Input: part model. Units: mm. Frame: model coordinates. Face numbers are marked on the shaded views. A direction names the side the tool comes from. Give positions to 0.01 mm unless a question says otherwise; leave off trailing zeros. Order: outer loops, then holes, each group sorted by start corner. A loop starts at its lowest first (then second) coordinate and runs counter-clockwise, first axis right, second up. Notation, with made-up numbers: (-18, 12) - (-7, 12) arc R16 cw to (-7, 31) - close; hole circle Ø10 at (30, -19.5). An arc over 180 degrees is marked (long way). Use a Markdown table: item, result.
from build123d import *

# Parameters (mm, degrees)
SKETCH_1_W           = 116
SKETCH_1_H           = 70
EXTRUDE_1_DEPTH      = 66
SKETCH_2_W           = 110
SKETCH_2_H           = 60
CUT_EXTRUDE_1_DEPTH  = 67
CUT_EXTRUDE_2_REACH  = 118
SKETCH_3_W           = 65
SKETCH_3_H           = 13
CUT_EXTRUDE_3_REACH  = 118
SKETCH_4_W           = 65
SKETCH_4_H           = 9.8
CUT_EXTRUDE_4_REACH  = 68
SKETCH_5_W           = 92
SKETCH_5_H           = 3
CUT_EXTRUDE_5_REACH  = 118
SKETCH_6_W           = 33
SKETCH_6_H           = 42
SKETCH_7_W           = 92
SKETCH_7_H           = 3
CUT_EXTRUDE_6_DEPTH  = 67
CUT_EXTRUDE_7_DEPTH  = 4
CUT_EXTRUDE_8_DEPTH  = 4
CUT_EXTRUDE_9_DEPTH  = 4
CUT_EXTRUDE_10_DEPTH = 4
CUT_EXTRUDE_11_DEPTH = 4
CUT_EXTRUDE_12_REACH = 118
CUT_EXTRUDE_13_DEPTH = 67
CUT_EXTRUDE_14_DEPTH = 67
CUT_EXTRUDE_15_DEPTH = 67
CUT_EXTRUDE_16_DEPTH = 67
CUT_EXTRUDE_17_DEPTH = 67
CUT_EXTRUDE_18_REACH = 68
CUT_EXTRUDE_19_REACH = 118
CUT_EXTRUDE_20_DEPTH = 67
FILLET_1_R           = 2
SKETCH_22_W          = 129.509915456
SKETCH_22_H          = 79.224014217
CUT_EXTRUDE_22_DEPTH = 30
SKETCH_23_W          = 92
SKETCH_23_H          = 66
CUT_EXTRUDE_23_DEPTH = 3
CUT_EXTRUDE_24_DEPTH = 8


with BuildPart() as part:
    # 스케치1 → 보스-돌출1 (new body)
    with BuildSketch(Plane.XZ.offset(33)):
        with Locations((0, 35)):
            Rectangle(SKETCH_1_W, SKETCH_1_H)
    extrude(amount=-EXTRUDE_1_DEPTH)

    # 스케치2 → 컷-돌출1 (cut)
    with BuildSketch(Plane.XY.offset(70)):
        Rectangle(SKETCH_2_W, SKETCH_2_H)
    extrude(amount=-CUT_EXTRUDE_1_DEPTH, mode=Mode.SUBTRACT)

    # 스케치3 → 컷-돌출2 (cut, up to next)
    with BuildSketch(Plane.ZY.offset(58), mode=Mode.PRIVATE) as cut_extrude_2_sk1:
        with Locations((37.5, 14.5)):
            Rectangle(SKETCH_3_W, SKETCH_3_H)
    cut_extrude_2_tool1 = extrude(cut_extrude_2_sk1.sketch, amount=-CUT_EXTRUDE_2_REACH, mode=Mode.PRIVATE) & part.part
    add(cut_extrude_2_tool1.solids().sort_by_distance((-58, 14.5, 37.5))[0], mode=Mode.SUBTRACT)

    # 스케치4 → 컷-돌출3 (cut, up to next)
    with BuildSketch(Plane.ZY.offset(58), mode=Mode.PRIVATE) as cut_extrude_3_sk1:
        with Locations((37.5, -16.3)):
            Rectangle(SKETCH_4_W, SKETCH_4_H)
    cut_extrude_3_tool1 = extrude(cut_extrude_3_sk1.sketch, amount=-CUT_EXTRUDE_3_REACH, mode=Mode.PRIVATE) & part.part
    add(cut_extrude_3_tool1.solids().sort_by_distance((-58, -16.3, 37.5))[0], mode=Mode.SUBTRACT)

    # 스케치5 → 컷-돌출4 (cut, up to next)
    with BuildSketch(Plane.XZ.offset(33), mode=Mode.PRIVATE) as cut_extrude_4_sk1:
        with Locations((0, 68.5)):
            Rectangle(SKETCH_5_W, SKETCH_5_H)
    cut_extrude_4_tool1 = extrude(cut_extrude_4_sk1.sketch, amount=-CUT_EXTRUDE_4_REACH, mode=Mode.PRIVATE) & part.part
    add(cut_extrude_4_tool1.solids().sort_by_distance((0, -33, 68.5))[0], mode=Mode.SUBTRACT)

    # 스케치6 → 컷-돌출5 (cut, up to next)
    with BuildSketch(Plane(origin=(58, 0, 0), x_dir=(0, 0, -1), z_dir=(1, 0, 0)), mode=Mode.PRIVATE) as cut_extrude_5_sk1:
        with Locations((-53.5, 0)):
            Rectangle(SKETCH_6_W, SKETCH_6_H)
    cut_extrude_5_tool1 = extrude(cut_extrude_5_sk1.sketch, amount=-CUT_EXTRUDE_5_REACH, mode=Mode.PRIVATE) & part.part
    add(cut_extrude_5_tool1.solids().sort_by_distance((58, 0, 53.5))[0], mode=Mode.SUBTRACT)

    # 스케치7 → 컷-돌출6 (cut, through all)
    with BuildSketch(Plane(origin=(0, 33, 0), x_dir=(-1, 0, 0), z_dir=(0, 1, 0))):
        with Locations((0, 68.5)):
            Rectangle(SKETCH_7_W, SKETCH_7_H)
    extrude(amount=-CUT_EXTRUDE_6_DEPTH, mode=Mode.SUBTRACT)

    # 스케치8 → 컷-돌출7 (cut, through all)
    with BuildSketch(Plane.XZ.offset(-30)):
        Polygon((-33.773502692, 35), (-30.886751346, 30), (-25.113248654, 30), (-22.226497308, 35), (-25.113248654, 40), (-30.886751346, 40), align=None)
    extrude(amount=-CUT_EXTRUDE_7_DEPTH, mode=Mode.SUBTRACT)

    # 스케치9 → 컷-돌출8 (cut, through all)
    with BuildSketch(Plane.XZ.offset(-30)):
        Polygon((-5.773502692, 35), (-2.886751346, 30), (2.886751346, 30), (5.773502692, 35), (2.886751346, 40), (-2.886751346, 40), align=None)
    extrude(amount=-CUT_EXTRUDE_8_DEPTH, mode=Mode.SUBTRACT)

    # 스케치10 → 컷-돌출9 (cut, through all)
    with BuildSketch(Plane.XZ.offset(-30)):
        Polygon((22.226497308, 35), (25.113248654, 30), (30.886751346, 30), (33.773502692, 35), (30.886751346, 40), (25.113248654, 40), align=None)
    extrude(amount=-CUT_EXTRUDE_9_DEPTH, mode=Mode.SUBTRACT)

    # 스케치11 → 컷-돌출10 (cut, through all)
    with BuildSketch(Plane.XZ.offset(-30)):
        Polygon((22.226497308, 15), (25.113248654, 10), (30.886751346, 10), (33.773502692, 15), (30.886751346, 20), (25.113248654, 20), align=None)
    extrude(amount=-CUT_EXTRUDE_10_DEPTH, mode=Mode.SUBTRACT)

    # 스케치12 → 컷-돌출11 (cut, through all)
    with BuildSketch(Plane.XZ.offset(-30)):
        Polygon((-5.773502692, 15), (-2.886751346, 10), (2.886751346, 10), (5.773502692, 15), (2.886751346, 20), (-2.886751346, 20), align=None)
    extrude(amount=-CUT_EXTRUDE_11_DEPTH, mode=Mode.SUBTRACT)

    # 스케치13 → 컷-돌출12 (cut, up to next)
    with BuildSketch(Plane(origin=(58, 0, 0), x_dir=(0, 0, -1), z_dir=(1, 0, 0)), mode=Mode.PRIVATE) as cut_extrude_12_sk1:
        Polygon((-23, -17.113248654), (-23, -22.886751346), (-18, -25.773502692), (-13, -22.886751346), (-13, -17.113248654), (-18, -14.226497308), align=None)
    cut_extrude_12_tool1 = extrude(cut_extrude_12_sk1.sketch, amount=-CUT_EXTRUDE_12_REACH, mode=Mode.PRIVATE) & part.part
    add(cut_extrude_12_tool1.solids().sort_by_distance((58, -20, 18))[0], mode=Mode.SUBTRACT)

    # 스케치14 → 컷-돌출13 (cut, through all)
    with BuildSketch(Plane.XZ.offset(33)):
        Polygon((-25.113248654, 40), (-30.886751346, 40), (-33.773502692, 35), (-30.886751346, 30), (-25.113248654, 30), (-22.226497308, 35), align=None)
    extrude(amount=-CUT_EXTRUDE_13_DEPTH, mode=Mode.SUBTRACT)

    # 스케치15 → 컷-돌출14 (cut, through all)
    with BuildSketch(Plane.XZ.offset(33)):
        Polygon((2.886751346, 40), (-2.886751346, 40), (-5.773502692, 35), (-2.886751346, 30), (2.886751346, 30), (5.773502692, 35), align=None)
    extrude(amount=-CUT_EXTRUDE_14_DEPTH, mode=Mode.SUBTRACT)

    # 스케치16 → 컷-돌출15 (cut, through all)
    with BuildSketch(Plane.XZ.offset(33)):
        Polygon((30.886751346, 40), (25.113248654, 40), (22.226497308, 35), (25.113248654, 30), (30.886751346, 30), (33.773502692, 35), align=None)
    extrude(amount=-CUT_EXTRUDE_15_DEPTH, mode=Mode.SUBTRACT)

    # 스케치17 → 컷-돌출16 (cut, through all)
    with BuildSketch(Plane.XZ.offset(33)):
        Polygon((30.886751346, 20), (25.113248654, 20), (22.226497308, 15), (25.113248654, 10), (30.886751346, 10), (33.773502692, 15), align=None)
    extrude(amount=-CUT_EXTRUDE_16_DEPTH, mode=Mode.SUBTRACT)

    # 스케치18 → 컷-돌출17 (cut, through all)
    with BuildSketch(Plane.XZ.offset(33)):
        Polygon((2.886751346, 20), (-2.886751346, 20), (-5.773502692, 15), (-2.886751346, 10), (2.886751346, 10), (5.773502692, 15), align=None)
    extrude(amount=-CUT_EXTRUDE_17_DEPTH, mode=Mode.SUBTRACT)

    # 스케치19 → 컷-돌출18 (cut, up to next)
    with BuildSketch(Plane.XZ.offset(33), mode=Mode.PRIVATE) as cut_extrude_18_sk1:
        Polygon((-25.113248654, 20), (-30.886751346, 20), (-33.773502692, 15), (-30.886751346, 10), (-25.113248654, 10), (-22.226497308, 15), align=None)
    cut_extrude_18_tool1 = extrude(cut_extrude_18_sk1.sketch, amount=-CUT_EXTRUDE_18_REACH, mode=Mode.PRIVATE) & part.part
    add(cut_extrude_18_tool1.solids().sort_by_distance((-28, -33, 15))[0], mode=Mode.SUBTRACT)

    # 스케치20 → 컷-돌출19 (cut, up to next)
    with BuildSketch(Plane(origin=(58, 0, 0), x_dir=(0, 0, -1), z_dir=(1, 0, 0)), mode=Mode.PRIVATE) as cut_extrude_19_sk1:
        Polygon((-18, 25.773502692), (-23, 22.886751346), (-23, 17.113248654), (-18, 14.226497308), (-13, 17.113248654), (-13, 22.886751346), align=None)
    cut_extrude_19_tool1 = extrude(cut_extrude_19_sk1.sketch, amount=-CUT_EXTRUDE_19_REACH, mode=Mode.PRIVATE) & part.part
    add(cut_extrude_19_tool1.solids().sort_by_distance((58, 20, 18))[0], mode=Mode.SUBTRACT)

    # 스케치21 → 컷-돌출20 (cut, through all)
    with BuildSketch(Plane(origin=(0, 33, 0), x_dir=(-1, 0, 0), z_dir=(0, 1, 0))):
        Polygon((22.226497308, 15), (25.113248654, 10), (30.886751346, 10), (33.773502692, 15), (30.886751346, 20), (25.113248654, 20), align=None)
    extrude(amount=-CUT_EXTRUDE_20_DEPTH, mode=Mode.SUBTRACT)

    # 필렛1
    fillet_1_edges = [part.edges().sort_by_distance(p)[0] for p in [
        (58, 33, 35),
        (-58, 33, 35),
        (58, -33, 35),
        (-58, -33, 35),
    ]]
    fillet(fillet_1_edges, radius=FILLET_1_R)

    # 스케치22 → 컷-돌출22 (cut)
    with BuildSketch(Plane.XY.offset(70)):
        with Locations((1.80270212, -0.616713883)):
            Rectangle(SKETCH_22_W, SKETCH_22_H)
    extrude(amount=-CUT_EXTRUDE_22_DEPTH, mode=Mode.SUBTRACT)

    # 스케치23 → 컷-돌출23 (cut)
    with BuildSketch(Plane.XY.offset(40)):
        Rectangle(SKETCH_23_W, SKETCH_23_H)
    extrude(amount=-CUT_EXTRUDE_23_DEPTH, mode=Mode.SUBTRACT)

    # 스케치24 → 컷-돌출24 (cut)
    with BuildSketch(Plane(origin=(58, 0, 0), x_dir=(0, 0, -1), z_dir=(1, 0, 0))):
        Polygon((-18, -14.226497308), (-18, 14.226497308), (-13, 20), (-2, 20), (-2, -20), (-13, -20), align=None)
    extrude(amount=-CUT_EXTRUDE_24_DEPTH, mode=Mode.SUBTRACT)


solid = part.part
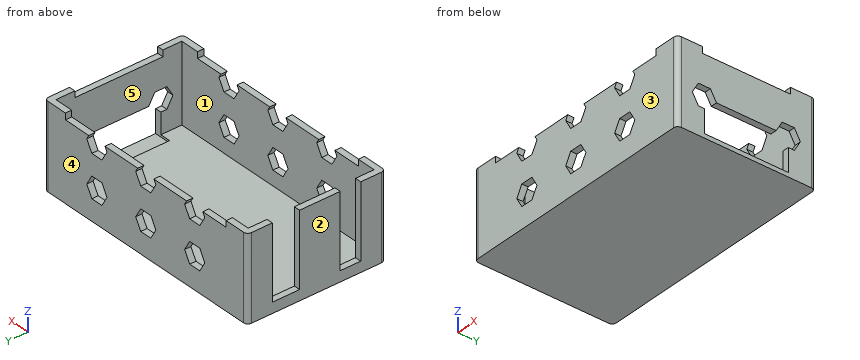
1. Material intervals for line 1 along Y through (x, z) = (-26, 6.5); line 2 along X through (y, z) = (4.5, 27); line 3 along Z through (x, y) = (-49.5, -1.5), sorted ascending.
Response:
| item | result |
|---|---|
| line 1 | y = -33 to -30, 30 to 33 |
| line 2 | x = -58 to -55, 55 to 58 |
| line 3 | z = 0 to 3 |
2. Section query B-B (y = 6). Return loops of the section in (x, z), then the cut area to 3 significant figures.
Response:
| item | result |
|---|---|
| outline | (-58, 0) - (58, 0) - (58, 2) - (50, 2) - (50, 3) - (-55, 3) - (-55, 40) - (-58, 40) - close; (55, 18) - (58, 18) - (58, 37) - (55, 37) - close |
| area | 508 mm^2 |
3. Section query C-C (x = 15.5). Return loops of the section in (y, z).
Response:
| item | result |
|---|---|
| outline | (-33, 0) - (33, 0) - (33, 37) - (30, 37) - (30, 3) - (-30, 3) - (-30, 37) - (-33, 37) - close |
4. Section query A-A (z = 7.5). Return loops of the section in (x, y), then the cut area to 3 significant figures.
Response:
| item | result |
|---|---|
| outline | (-58, -31) arc R2 ccw to (-56, -33) - (56, -33) arc R2 ccw to (58, -31) - (58, -20) - (55, -20) - (55, -30) - (-55, -30) - (-55, -21.2) - (-58, -21.2) - close; (-58, -11.4) - (-55, -11.4) - (-55, 8) - (-58, 8) - close; (-58, 21) - (-55, 21) - (-55, 30) - (55, 30) - (55, 20) - (58, 20) - (58, 31) arc R2 ccw to (56, 33) - (-56, 33) arc R2 ccw to (-58, 31) - close |
| area | 864 mm^2 |
5. Pin query (flat end, axial travel): pin 1 (3 mm diameter, centred on y = 17, z = 16.5, fed in from -X); pin 2 (1.5 mm diameter, centred on x = 57, z = 38, fed in from +Y); pin 3 (2.5 mm diameter, centred on x = 27, y = -31.5, fed in from +Z); pin 4 (2.5 mm diameter, centred on x = 15.5, y = -31.5, fed in from +Z). Return the tip coordinate at first contact, or that it passes through.
Response:
| item | result |
|---|---|
| pin 1 | passes through |
| pin 2 | stops at y = 32.98 |
| pin 3 | stops at z = 30 |
| pin 4 | stops at z = 37 |
6. Set-up query: the marked faces 4 and 5. Return all of +Z, -Z, +X, -X, +Y, -Y with unobstructed straight access to the full face (end or side cutting, diameter ignored); none if empty.
Response:
| item | result |
|---|---|
| face 4 | +Z, -Z, +X, -X, +Y |
| face 5 | +Z |
7. Section query D-D (y = 28). Return loops of the section in (x, z).
Response:
| item | result |
|---|---|
| outline | (-58, 0) - (58, 0) - (58, 40) - (55, 40) - (55, 3) - (-55, 3) - (-55, 40) - (-58, 40) - close |
8. Mould query, pull axis Y, two halves, no side actions, for the marked faces 1, 2 and 3. Classes: pulls with the +Y half, pulls with the -Y half, needs draft (parallel to the pull), parting line crosses it, or undercut.
Response:
| item | result |
|---|---|
| face 1 | undercut |
| face 2 | needs draft |
| face 3 | pulls with the -Y half |
